Input: dimensioned drawing with shaded views. Units: mm. Origin: part minimum x, y, z. Give positions to 0.01 mm unless a question says otherwise; leave off trailing zeros. Loops run counter-clockwise (first coordinate to the right, second up) from the corner with the lowest first, then second, coordinate; pieces in that order, holes last.
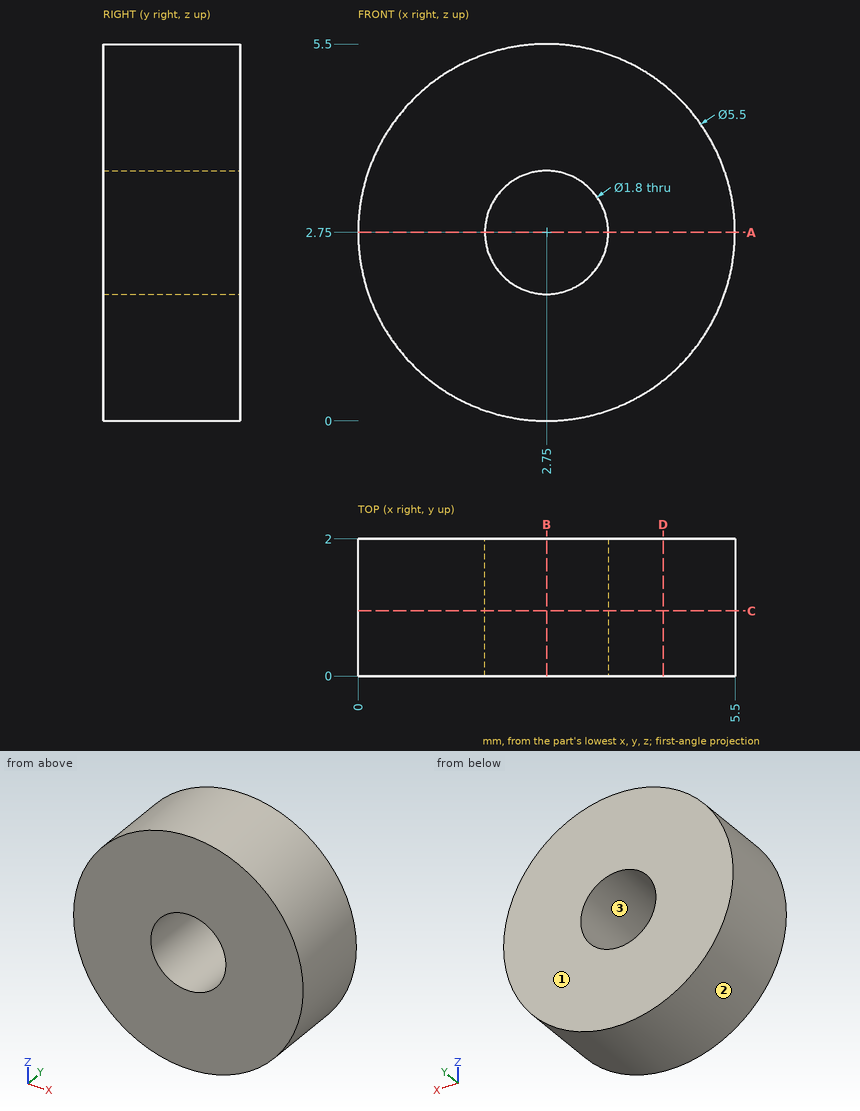
(1) Section C-C, the plane y = 0.95. Return the cut outline in (x, z).
A:
outline: circle Ø5.5 at (2.75, 2.75); hole circle Ø1.8 at (2.75, 2.75)
(2) First-contact query: pin 1 (1 mm diameter, centred on x = 4, y = 1.5, fed in from +Z). Flat tip, straight axial feed; report the tip coordinate or a pass-through.
A:
pin 1: stops at z = 5.4
(3) Ray query, line 1 along Z through (x, y) = (2.75, 0.6); line 2 along Z through (x, y) = (2.25, 0.8); line 3 along X through (y, z) = (1.4, 3.4). Return the intervals inside material, ascending.
A:
line 1: z = 0 to 1.85, 3.65 to 5.5
line 2: z = 0.05 to 2, 3.5 to 5.45
line 3: x = 0.08 to 2.13, 3.37 to 5.42
(4) Section D-D, the plane x = 4.45. Return the cut outline in (y, z).
A:
outline: (0, 0.59) - (2, 0.59) - (2, 4.91) - (0, 4.91) - close
(5) Section B-B, the plane x = 2.75. Return the cut outline in (y, z), then the cut area to 3 significant figures.
A:
outline: (0, 0) - (2, 0) - (2, 1.85) - (0, 1.85) - close; (0, 3.65) - (2, 3.65) - (2, 5.5) - (0, 5.5) - close
area: 7.40 mm2
(6) Section A-A, the plane z = 2.75. Return the cut outline in (x, y), then the cut area to 3 significant figures.
A:
outline: (0, 0) - (1.85, 0) - (1.85, 2) - (0, 2) - close; (3.65, 0) - (5.5, 0) - (5.5, 2) - (3.65, 2) - close
area: 7.40 mm2
(7) Mould query, pull axis X, two halves, no side actions, for the marked faces 1, 2 and 3. Classes: pulls with the +X half, pulls with the -X half, needs draft (parallel to the pull), parting line crosses it, or undercut.
A:
face 1: needs draft
face 2: parting line crosses it
face 3: undercut
